from build123d import *

# Parameters (mm, degrees)
BASEPLATE_OUTLINE_R = 2.1
BASEPLATE_DEPTH     = 2.8
CUT_EXTRUDE1_REACH  = 115.438
SKETCH3_W           = 15.4
SKETCH3_H           = 19.2
SKETCH3_W_2         = 15.6
SKETCH3_W_3         = 16.2
SKETCH3_H_2         = 24.9
CUT_EXTRUDE2_REACH  = 115.438
FILLET1_R           = 5


# Read off the part's stored shape, not the designer's step: BasePlate
with BuildPart() as part:
    # BasePlate outline → BasePlate (new body)
    with BuildSketch(Plane(origin=(0, 0, 0), x_dir=(1, 0, 0), z_dir=(0, 1, 0))):
        with BuildLine():
            Line((43.502626614, -5.852332608), (48.792614178, -5.852332608))
            ThreePointArc((48.792614178, -5.852332608), (49.082078508, -5.760021707), (49.264659986, -5.517174213))
            Line((49.264659986, -5.517174213), (50.078201202, -3.187491002))
            ThreePointArc((50.078201202, -3.187491002), (50.26078268, -2.944643509), (50.55024701, -2.852332608))
            Line((50.55024701, -2.852332608), (58.116695703, -2.852332608))
            ThreePointArc((58.116695703, -2.852332608), (58.484685739, -3.013831008), (58.614956567, -3.393999275))
            ThreePointArc((58.614956567, -3.393999275), (64.799237397, -7.61016844), (65.229166667, -0.137781095))
            ThreePointArc((65.229166667, -0.137781095), (65.061014427, 0.043158816), (65, 0.282515593))
            Line((65, 0.282515593), (65, 83.012819192))
            ThreePointArc((65, 83.012819192), (65.061014427, 83.252175969), (65.229166667, 83.433115879))
            ThreePointArc((65.229166667, 83.433115879), (65.940559159, 90.088226551), (59.285448487, 89.376834059))
            ThreePointArc((59.285448487, 89.376834059), (59.104508577, 89.208681819), (58.8651518, 89.147667392))
            Line((58.8651518, 89.147667392), (6.1348482, 89.147667392))
            ThreePointArc((6.1348482, 89.147667392), (5.895491423, 89.208681819), (5.714551513, 89.376834059))
            ThreePointArc((5.714551513, 89.376834059), (-0.940559159, 90.088226551), (-0.229166667, 83.433115879))
            ThreePointArc((-0.229166667, 83.433115879), (-0.061014427, 83.252175969), (0, 83.012819192))
            Line((0, 83.012819192), (0, 0.282515593))
            ThreePointArc((0, 0.282515593), (-0.061014427, 0.043158816), (-0.229166667, -0.137781095))
            ThreePointArc((-0.229166667, -0.137781095), (0.200762603, -7.61016844), (6.385043433, -3.393999275))
            ThreePointArc((6.385043433, -3.393999275), (6.515314261, -3.013831008), (6.883304297, -2.852332608))
            Line((6.883304297, -2.852332608), (14.44975299, -2.852332608))
            ThreePointArc((14.44975299, -2.852332608), (14.73921732, -2.944643509), (14.921798798, -3.187491002))
            Line((14.921798798, -3.187491002), (15.735340014, -5.517174213))
            ThreePointArc((15.735340014, -5.517174213), (15.917921492, -5.760021707), (16.207385822, -5.852332608))
            Line((16.207385822, -5.852332608), (21.497373386, -5.852332608))
            ThreePointArc((21.497373386, -5.852332608), (21.786837716, -5.760021707), (21.969419194, -5.517174213))
            Line((21.969419194, -5.517174213), (22.78296041, -3.187491002))
            ThreePointArc((22.78296041, -3.187491002), (22.965541888, -2.944643509), (23.255006218, -2.852332608))
            Line((23.255006218, -2.852332608), (41.744993782, -2.852332608))
            ThreePointArc((41.744993782, -2.852332608), (42.034458112, -2.944643509), (42.21703959, -3.187491002))
            Line((42.21703959, -3.187491002), (43.030580806, -5.517174213))
            ThreePointArc((43.030580806, -5.517174213), (43.213162284, -5.760021707), (43.502626614, -5.852332608))
        make_face()
        with Locations((2.1, -3.752332608)):
            Circle(BASEPLATE_OUTLINE_R, mode=Mode.SUBTRACT)
        with Locations((62.9, -3.752332608)):
            Circle(BASEPLATE_OUTLINE_R, mode=Mode.SUBTRACT)
        with Locations((2.1, 87.047667392)):
            Circle(BASEPLATE_OUTLINE_R, mode=Mode.SUBTRACT)
        with Locations((62.9, 87.047667392)):
            Circle(BASEPLATE_OUTLINE_R, mode=Mode.SUBTRACT)
    extrude(amount=BASEPLATE_DEPTH)

    # Sketch3 → Cut-Extrude1 (cut, up to next)
    with BuildSketch(Plane(origin=(0, 2.8, 0), x_dir=(1, 0, 0), z_dir=(0, 1, 0)), mode=Mode.PRIVATE) as cut_extrude1_sk1:
        Polygon((4.8, 1.147667392), (49.5, 1.147667392), (49.5, 24.447667392), (63, 24.447667392), (63, 22.647667392), (65, 22.647667392), (65, 42.047667392), (63, 42.047667392), (63, 40.047667392), (35.4, 40.047667392), (35.4, 61.647667392), (33.1, 61.647667392), (33.1, 66.147667392), (19.8, 66.147667392), (19.8, 61.647667392), (4.8, 61.647667392), align=None)
    cut_extrude1_tool1 = extrude(cut_extrude1_sk1.sketch, amount=-CUT_EXTRUDE1_REACH, mode=Mode.PRIVATE) & part.part
    # Sketch3 → Cut-Extrude1 (cut, up to next)
    with BuildSketch(Plane(origin=(0, 2.8, 0), x_dir=(1, 0, 0), z_dir=(0, 1, 0)), mode=Mode.PRIVATE) as cut_extrude1_sk2:
        Polygon((55.9, 6.647667392), (63, 6.647667392), (63, 4.147667392), (65, 4.147667392), (65, 16.747667392), (63, 16.747667392), (63, 14.947667392), (55.9, 14.947667392), align=None)
    cut_extrude1_tool2 = extrude(cut_extrude1_sk2.sketch, amount=-CUT_EXTRUDE1_REACH, mode=Mode.PRIVATE) & part.part
    # Sketch3 → Cut-Extrude1 (cut, up to next)
    with BuildSketch(Plane(origin=(0, 2.8, 0), x_dir=(1, 0, 0), z_dir=(0, 1, 0)), mode=Mode.PRIVATE) as cut_extrude1_sk3:
        with Locations((14, 79.547667392)):
            Rectangle(SKETCH3_W, SKETCH3_H)
    cut_extrude1_tool3 = extrude(cut_extrude1_sk3.sketch, amount=-CUT_EXTRUDE1_REACH, mode=Mode.PRIVATE) & part.part
    # Sketch3 → Cut-Extrude1 (cut, up to next)
    with BuildSketch(Plane(origin=(0, 2.8, 0), x_dir=(1, 0, 0), z_dir=(0, 1, 0)), mode=Mode.PRIVATE) as cut_extrude1_sk4:
        with Locations((32, 79.547667392)):
            Rectangle(SKETCH3_W_2, SKETCH3_H)
    cut_extrude1_tool4 = extrude(cut_extrude1_sk4.sketch, amount=-CUT_EXTRUDE1_REACH, mode=Mode.PRIVATE) & part.part
    # Sketch3 → Cut-Extrude1 (cut, up to next)
    with BuildSketch(Plane(origin=(0, 2.8, 0), x_dir=(1, 0, 0), z_dir=(0, 1, 0)), mode=Mode.PRIVATE) as cut_extrude1_sk5:
        with Locations((51, 76.697667392)):
            Rectangle(SKETCH3_W_3, SKETCH3_H_2)
    cut_extrude1_tool5 = extrude(cut_extrude1_sk5.sketch, amount=-CUT_EXTRUDE1_REACH, mode=Mode.PRIVATE) & part.part
    add(cut_extrude1_tool1.solids().sort_by_distance((28.204461, 2.8, -30.008726))[0], mode=Mode.SUBTRACT)
    add(cut_extrude1_tool2.solids().sort_by_distance((60.812891, 2.8, -10.69283))[0], mode=Mode.SUBTRACT)
    add(cut_extrude1_tool3.solids().sort_by_distance((14, 2.8, -79.547667))[0], mode=Mode.SUBTRACT)
    add(cut_extrude1_tool4.solids().sort_by_distance((32, 2.8, -79.547667))[0], mode=Mode.SUBTRACT)
    add(cut_extrude1_tool5.solids().sort_by_distance((51, 2.8, -76.697667))[0], mode=Mode.SUBTRACT)

    # Sketch4 → Cut-Extrude2 (cut, up to next)
    with BuildSketch(Plane(origin=(0, 2.8, 0), x_dir=(1, 0, 0), z_dir=(0, 1, 0)), mode=Mode.PRIVATE) as cut_extrude2_sk1:
        Polygon((65, 59.347667392), (63, 59.347667392), (63, 57.347667392), (40.2, 57.347667392), (40.2, 47.947667392), (38.3, 47.947667392), (38.3, 42.447667392), (60.9, 42.447667392), (60.9, 50.047667392), (63, 50.047667392), (63, 48.047667392), (65, 48.047667392), align=None)
    cut_extrude2_tool1 = extrude(cut_extrude2_sk1.sketch, amount=-CUT_EXTRUDE2_REACH, mode=Mode.PRIVATE) & part.part
    add(cut_extrude2_tool1.solids().sort_by_distance((51.560754, 2.8, -50.163969))[0], mode=Mode.SUBTRACT)

    # Fillet1
    fillet1_edges = [part.edges().sort_by_distance(p)[0] for p in [
        (49.5, 1.4, -24.447667392),
    ]]
    fillet(fillet1_edges, radius=FILLET1_R)


solid = part.part
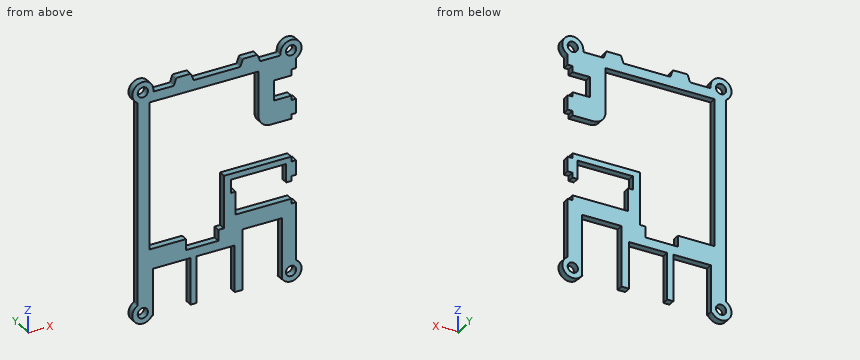
Design review of the part built by this model. Coordinates are the model's own, in mm. Round coordinates to 2 decimals unless told otherwise and drop trailing zeros. Order: outer loops, then holes, each group sorted by start corner. A loop starts at its lowest first (then second) coordinate and runs counter-clockwise, first axis right, second up. Notation, with made-up numbers: M 80,18 L 105,18 A9 ccw 105,23 Z; hole C 5.5,64 d4. An arc over 180 degrees is marked long. Answer as CSV lines item,"result". Start each with the question number.
1) Add section D-D (x = 45.5). Give the boundary of the cut face in (y, z).
2) Add section C-C (x = 2.1). Give the boundary of the cut face in (y, z), then the cut area to 3 significant figures.
3) For pin 1 Ø1.4 at (x, y) = (60, 1) entering from -Z; pin 2 Ø1.5 at (y, z) = (2, -15.5) entering from -X; pin 3 Ø0.8 at (x, y) = (29.5, 1.5) entering from +Z, all flat-tipped, find the tip position at first contact; note any pin that passes through.
4) Wall thickness on line 1 along Z through (x, y) = (62.9, 0.85); line 2 along Z through (x, y) = (48.5, 1.9); line 3 along X through (y, z) = (2.6, -77.5): over which ranges is each line inside the solid? List them lowest first. Write a range as [from, to].
5) Add section B-B (z = -11.5). Give the boundary of the cut face in (x, y).
6) Add section A-A (x = 30.5). Give the boundary of the cut face in (y, z).
Resolved:
1,outline,"M 0,-64.25 L 2.8,-64.25 L 2.8,-57.35 L 0,-57.35 Z; M 0,-42.45 L 2.8,-42.45 L 2.8,-40.05 L 0,-40.05 Z; M 0,-1.15 L 2.8,-1.15 L 2.8,5.85 L 0,5.85 Z"
2,outline,"M 0,-91.35 L 2.8,-91.35 L 2.8,-89.15 L 0,-89.15 Z; M 0,-84.95 L 2.8,-84.95 L 2.8,1.65 L 0,1.65 Z; M 0,5.85 L 2.8,5.85 L 2.8,8.05 L 0,8.05 Z"
2,area,"255 mm^2"
3,pin 1,"z = -90.74"
3,pin 2,"x = 0"
3,pin 3,"z = 2.85"
4,line 1,"[-91.35, -89.15], [-84.95, -57.35], [-50.05, -40.05], [-24.45, -14.95], [-6.65, 1.65], [5.85, 8.05]"
4,line 2,"[-64.25, -57.35], [-42.45, -40.05], [-1.15, 5.85]"
4,line 3,"[0, 6.3], [21.7, 24.2], [39.8, 42.9], [59.1, 65]"
5,outline,"M 0,0 L 4.8,0 L 4.8,2.8 L 0,2.8 Z; M 49.5,0 L 55.9,0 L 55.9,2.8 L 49.5,2.8 Z"
6,outline,"M 0,-69.95 L 2.8,-69.95 L 2.8,-66.15 L 0,-66.15 Z; M 0,-1.15 L 2.8,-1.15 L 2.8,2.85 L 0,2.85 Z"
